from build123d import *

# Parameters (mm, degrees)
SKETCH1_W                = 110.49
SKETCH1_H                = 80.01
BOSS_EXTRUDE1_DEPTH      = 33.909
SKETCH2_W                = 12.446
SKETCH2_H                = 78.486
CUT_EXTRUDE1_DEPTH       = 13.208
SKETCH3_W                = 8.89
SKETCH3_H                = 19.177
CUT_EXTRUDE2_DEPTH       = 12.446
CUT_EXTRUDE5_DEPTH       = 5.08
CUT_EXTRUDE3_REACH       = 104.973
SKETCH4_R                = 1.7145
SKETCH5_R                = 1.7145
CUT_EXTRUDE4_DEPTH       = 77.172372492
SKETCH8_R                = 3.175
BOSS_EXTRUDE2_DEPTH      = 2.54
LPATTERN1_COUNT          = 6
LPATTERN1_PITCH          = 8.89
M3_CLEARANCE_HOLE1_D     = 3.4
M3_CLEARANCE_HOLE1_DEPTH = 2.999994
M3_CLEARANCE_HOLE1_TIP   = 1.021463052


with BuildPart() as part:
    # Sketch1 → Boss-Extrude1 (new body)
    with BuildSketch(Plane(origin=(0, 0, 0), x_dir=(1, 0, 0), z_dir=(0, 1, 0))):
        Rectangle(SKETCH1_W, SKETCH1_H)
    extrude(amount=BOSS_EXTRUDE1_DEPTH)

    # Sketch2 → Cut-Extrude1 (cut)
    with BuildSketch(Plane(origin=(0, 33.909, 0), x_dir=(1, 0, 0), z_dir=(0, 1, 0))):
        with Locations((49.022, -0.762)):
            Rectangle(SKETCH2_W, SKETCH2_H)
    extrude(amount=-CUT_EXTRUDE1_DEPTH, mode=Mode.SUBTRACT)

    # Sketch3 → Cut-Extrude2 (cut)
    with BuildSketch(Plane(origin=(55.245, 0, 0), x_dir=(0, 0, -1), z_dir=(1, 0, 0))):
        with Locations((34.036, 11.1125)):
            Rectangle(SKETCH3_W, SKETCH3_H)
    extrude(amount=-CUT_EXTRUDE2_DEPTH, mode=Mode.SUBTRACT)

    # Sketch6 → Cut-Extrude5 (cut)
    with BuildSketch(Plane.ZY.offset(55.245)):
        Polygon((-38.481, 33.909), (40.005, 33.909), (40.005, 1.524), (29.845, 1.524), (29.845, 13.462), (-38.481, 13.462), align=None)
    extrude(amount=-CUT_EXTRUDE5_DEPTH, mode=Mode.SUBTRACT)

    # Sketch4 → Cut-Extrude3 (cut, up to next)
    with BuildSketch(Plane(origin=(0, 0, -40.005), x_dir=(-1, 0, 0), z_dir=(0, 0, -1)), mode=Mode.PRIVATE) as cut_extrude3_sk1:
        with Locations((-49.4157, 24.9047)):
            Circle(SKETCH4_R)
    cut_extrude3_tool1 = extrude(cut_extrude3_sk1.sketch, amount=-CUT_EXTRUDE3_REACH, mode=Mode.PRIVATE) & part.part
    # Sketch4 → Cut-Extrude3 (cut, up to next)
    with BuildSketch(Plane(origin=(0, 0, -40.005), x_dir=(-1, 0, 0), z_dir=(0, 0, -1)), mode=Mode.PRIVATE) as cut_extrude3_sk2:
        with BuildLine():
            Line((51.816, 26.543), (55.245, 26.543))
            Line((55.245, 26.543), (55.245, 23.2918))
            Line((55.245, 23.2918), (51.816, 23.2918))
            ThreePointArc((51.816, 23.2918), (50.1904, 24.9174), (51.816, 26.543))
        make_face()
    cut_extrude3_tool2 = extrude(cut_extrude3_sk2.sketch, amount=-CUT_EXTRUDE3_REACH, mode=Mode.PRIVATE) & part.part
    add(cut_extrude3_tool1.solids().sort_by_distance((49.4157, 24.9047, -40.005))[0], mode=Mode.SUBTRACT)
    add(cut_extrude3_tool2.solids().sort_by_distance((-52.878141, 24.9174, -40.005))[0], mode=Mode.SUBTRACT)

    # Sketch5 → Cut-Extrude4 (cut, through all)
    with BuildSketch(Plane(origin=(0, 0, 0), x_dir=(-1, 0, 0), z_dir=(0, -1, 0))):
        with Locations(Location((-50.3936, 34.3281, 0), (0, 0, 90))):
            Circle(SKETCH5_R)
        with BuildLine():
            Line((51.816, -35.2806), (55.245, -35.2806))
            Line((55.245, -35.2806), (55.245, -32.1056))
            Line((55.245, -32.1056), (51.816, -32.1056))
            ThreePointArc((51.816, -32.1056), (50.2285, -33.6931), (51.816, -35.2806))
        make_face()
    extrude(amount=-CUT_EXTRUDE4_DEPTH, mode=Mode.SUBTRACT)

    # Sketch8 → Boss-Extrude2 (add)
    with BuildSketch(Plane(origin=(0, 20.701, 0), x_dir=(1, 0, 0), z_dir=(0, 1, 0))):
        with Locations(Location((49.022, 20.701, 0), (0, 0, 270))):
            Circle(SKETCH8_R)
    boss_extrude2 = extrude(amount=BOSS_EXTRUDE2_DEPTH)

    # LPattern1: Boss-Extrude2 ×6
    with Locations(*[(0, 0, i * LPATTERN1_PITCH) for i in range(1, LPATTERN1_COUNT)]):
        add(boss_extrude2)

    # M3 Clearance Hole1
    with Locations(Plane(origin=(0, 0, 0), x_dir=(-1, 0, 0), z_dir=(0, -1, 0))):
        with Locations((-39.8936, -12.6719), (20.1064, -12.6719)):
            Hole(M3_CLEARANCE_HOLE1_D / 2, depth=M3_CLEARANCE_HOLE1_DEPTH)
            with Locations((0, 0, -(M3_CLEARANCE_HOLE1_DEPTH + M3_CLEARANCE_HOLE1_TIP / 2))):  # 118° drill point
                Cone(0, M3_CLEARANCE_HOLE1_D / 2, M3_CLEARANCE_HOLE1_TIP, mode=Mode.SUBTRACT)


solid = part.part
Design review of the part built by this model. Coordinates are the model's own, in mm. A direction names the side the tool comes from. Give positions to 0.01 mm unless a question says otherwise; leave off trailing zeros. Loops run counter-clockwise (first coordinate to the right, second up) from the corner with the lowest first, then second, coordinate; pieces in that order, holes last. Notation, with made-up numbers: (7, 25.5) -> (25, 25.5) arc R24 cw to (25, 56.5) -> close; hole circle Ø7 at (14, 46.5). An arc over 180 degrees is marked (long way). One line per question, with ' | ' between items. Start each with the question number.
(1) We need section B-B (z = -27). State the section outline as (x, y) points (3 decimals), and give its area (3 significant figures).
(2) For line 1 (X direction, y = 2.5, z = 14) (3 decimals); line 2 (X direction, y = 28.5, z = 2) (3 decimals); line 3 (X direction, y = 20, z = 21) (3 decimals), list the stretches that pass through material, from the lowest coordinate up.
(3) We need section A-A (y = 8.5). State the section outline as (x, z) points (3 decimals), and give its area (3 significant figures).
(4) We need section C-C (y = 28.5). State the section outline as (x, z) points (3 decimals), and give its area (3 significant figures).
(5) Insertion check: P1, Ø5, axis at x = 49, z = -3.5, coming from the +Y side; P2, Ø3.5, axis at x = 47, y = 23.5, coming from the +Z side; P3, Ø2.5, axis at x = -52, z = -17.5, coming from the +Y side. Each pin has a flat end and moves straight along its axis. Give the tip position at first contact, or say it passes through.
(6) For faces 4 (the face through (45.923, 21.953, -3.609)), 5 (the face through (49, 18, -38.481)), 6 (the face through (-53, 1.524, 36)), list the 3-axis set-ups (+Z, -Z, +X, -X, +Y, -Y) from which the entire face can be reached by the end or side of a thin tool; tool diameter is ignored.
(7) We need section D-D (y = 15). State the section outline as (x, z) points (3 decimals).
(8) Draft analysis for pull direction Z (two halves, no side actions). For faces 1 (the face through (-53, 21, -38.481)), 2 (the face through (42.799, 25, 1)), 3 (the face through (-53, 13.462, -4)), state which applies: +Z half, -Z half, draft (parallel to the pull), parting line (faces both ways), or undercut.
The answers:
1) outline: (-55.245, 0) -> (55.245, 0) -> (55.245, 20.701) -> (42.799, 20.701) -> (42.799, 33.909) -> (-50.165, 33.909) -> (-50.165, 13.462) -> (-55.245, 13.462) -> close | area: 3,480 mm^2
2) line 1: x = -55.245 to -21.168, -19.045 to 38.832, 40.955 to 55.245 | line 2: x = -50.165 to 42.799 | line 3: x = -50.165 to 55.245
3) outline: (-55.245, -40.005) -> (55.245, -40.005) -> (55.245, -38.481) -> (42.799, -38.481) -> (42.799, -29.591) -> (55.245, -29.591) -> (55.245, 40.005) -> (-50.165, 40.005) -> (-50.165, 29.845) -> (-55.245, 29.845) -> close | area: 8,680 mm^2
4) outline: (-55.245, -40.005) -> (55.245, -40.005) -> (55.245, -38.481) -> (42.799, -38.481) -> (42.799, 40.005) -> (-50.165, 40.005) -> (-50.165, -38.481) -> (-55.245, -38.481) -> close | area: 7,460 mm^2
5) P1: stops at y = 23.24 | P2: stops at z = 26.91 | P3: stops at y = 13.46
6) face 4: +Y | face 5: +X, +Y | face 6: +Z, -X, +Y
7) outline: (-55.245, -40.005) -> (55.245, -40.005) -> (55.245, -38.481) -> (42.799, -38.481) -> (42.799, -29.591) -> (55.245, -29.591) -> (55.245, 40.005) -> (-50.165, 40.005) -> (-50.165, -38.481) -> (-55.245, -38.481) -> close
8) face 1: +Z half | face 2: undercut | face 3: draft
